Part print with two shaded views. Sizes in mm from the minimum x, y, z corner. Round coordinates to 2 decimals unless told otherwise and drop trailing zeros. Write each loop counter-clockwise with the first axis right and the second up, starting at its lowest first coordinate (ties: lowest second). Pieces come first, ordered by that corner, then holes. Notation, with made-up numbers: (9.5, 89.5) -> (22.5, 89.5) arc R25 cw to (22.5, 128.5) -> close; hole circle Ø11 at (-12.75, -13.5). An arc over 180 degrees is marked (long way). Answer as CSV lines item,"result".
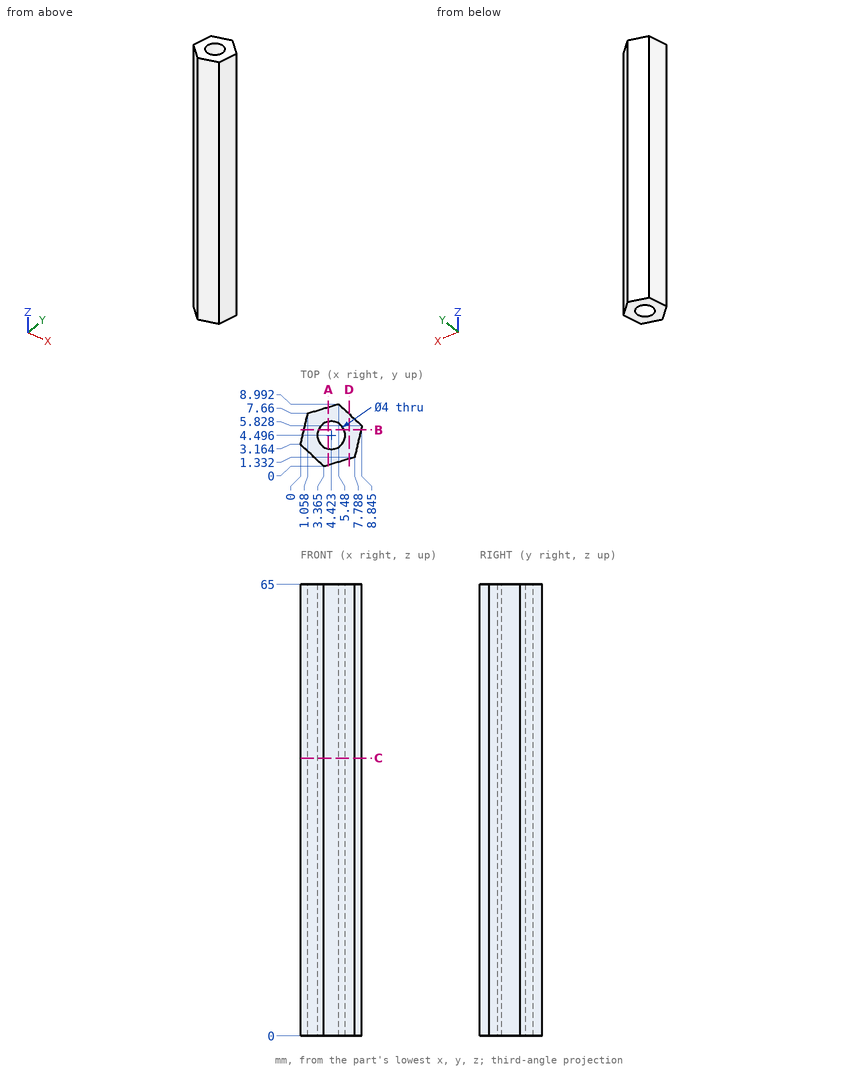
1. Probe line 1 along X through (y, z) = (4, 53) (1 decimal); line 2 along Y through (x, z) = (2.75, 55.5) (1 decimal); line 3 along Y through (x, z) = (4.5, 27) (1 decimal). List the from-to ranges inside material, lowest first.
Results found:
line 1,"x = 0.2 to 2.5, 6.4 to 8.4"
line 2,"y = 0.6 to 3.4, 5.6 to 8.2"
line 3,"y = 0.3 to 2.5, 6.5 to 8.7"
2. Cut at B-B, the plane y = 5.25. Write the cut outline in (x, z) (1 decimal).
Results found:
outline,"(0.5, 0) -> (2.6, 0) -> (2.6, 65) -> (0.5, 65) -> close; (6.3, 0) -> (8.7, 0) -> (8.7, 65) -> (6.3, 65) -> close"
3. Cut at D-D, the plane x = 7. Write the cut outline in (y, z) (1 decimal).
Results found:
outline,"(1.1, 0) -> (7.6, 0) -> (7.6, 65) -> (1.1, 65) -> close"
4. Cut at A-A, the plane x = 4. Write the cut outline in (y, z), then the cut area to 3 significant figures.
Results found:
outline,"(0.19, 0) -> (2.54, 0) -> (2.54, 65) -> (0.19, 65) -> close; (6.45, 0) -> (8.55, 0) -> (8.55, 65) -> (6.45, 65) -> close"
area,"289 mm2"
5. Cut at C-C, the plane z = 40. Write the cut outline in (x, y) (1 decimal).
Results found:
outline,"(0, 3.2) -> (3.4, 0) -> (7.8, 1.3) -> (8.8, 5.8) -> (5.5, 9) -> (1.1, 7.7) -> close; hole circle Ø4 at (4.4, 4.5)"
6. Drop flat-ended pins along their axis: pin 1 Ø1 at (y, z) = (6.5, 40) entering from +X; pin 2 Ø1.5 at (x, z) = (4.5, 35.5) entering from -Y (1 decimal); pin 3 Ø2 at (y, z) = (6.5, 44) entering from -X. Give the stop position or say it passes through.
Results found:
pin 1,"stops at x = 8.66"
pin 2,"stops at y = 0.1"
pin 3,"stops at x = 0.55"
